```python
from build123d import *

# Parameters (mm, degrees)
SKICA1_R                 = 16.78
P_IDAT_VYSUNUT_M1_DEPTH  = 50.7
SKICA2_R                 = 5.65
P_IDAT_VYSUNUT_M2_DEPTH  = 4.61
SKICA3_R                 = 1.565
P_IDAT_VYSUNUT_M3_DEPTH  = 8.5
SKETCH6_R                = 23.5
BOSS_EXTRUDE1_DEPTH      = 3
SKETCH8_W                = 4.15
SKETCH8_H                = 3
SKETCH8_W_2              = 3
SKETCH8_H_2              = 4.15
ODEBRAT_VYSUNUT_M2_DEPTH = 3


with BuildPart() as part:
    # Skica1 → Přidat vysunutím1 (new body)
    with BuildSketch(Plane(origin=(0, 0, 0), x_dir=(1, 0, 0), z_dir=(0, 1, 0))):
        with Locations(Location((0, 0, 0), (0, 0, 90))):
            Circle(SKICA1_R)
    extrude(amount=P_IDAT_VYSUNUT_M1_DEPTH)

    # Skica2 → Přidat vysunutím2 (add)
    with BuildSketch(Plane(origin=(0, 50.7, 0), x_dir=(1, 0, 0), z_dir=(0, 1, 0))):
        with Locations(Location((0, 0, 0), (0, 0, 270))):
            Circle(SKICA2_R)
    extrude(amount=P_IDAT_VYSUNUT_M2_DEPTH)

    # Skica3 → Přidat vysunutím3 (add)
    with BuildSketch(Plane(origin=(0, 55.31, 0), x_dir=(1, 0, 0), z_dir=(0, 1, 0))):
        with Locations(Location((0, 0, 0), (0, 0, 270))):
            Circle(SKICA3_R)
    extrude(amount=P_IDAT_VYSUNUT_M3_DEPTH)

    # Sketch6 → Boss-Extrude1 (add)
    with BuildSketch(Plane.XZ):
        with Locations(Location((0, 0, 0), (0, 0, 270))):
            Circle(SKETCH6_R)
    extrude(amount=BOSS_EXTRUDE1_DEPTH)

    # Sketch8 → Odebrat vysunutím2 (cut)
    with BuildSketch(Plane(origin=(0, 0, 0), x_dir=(1, 0, 0), z_dir=(0, 1, 0))):
        with Locations((20.075, 0)):
            Rectangle(SKETCH8_W, SKETCH8_H)
        Polygon((11.66726189, -13.788582233), (14.601755032, -16.723075375), (16.723075375, -14.601755032), (13.788582233, -11.66726189), align=None)
        with Locations((0, -20.075)):
            Rectangle(SKETCH8_W_2, SKETCH8_H_2)
        Polygon((-13.788582233, -11.66726189), (-16.723075375, -14.601755032), (-14.601755032, -16.723075375), (-11.66726189, -13.788582233), align=None)
        with Locations((-20.075, 0)):
            Rectangle(SKETCH8_W, SKETCH8_H)
        Polygon((-11.66726189, 13.788582233), (-14.601755032, 16.723075375), (-16.723075375, 14.601755032), (-13.788582233, 11.66726189), align=None)
        with Locations((0, 20.075)):
            Rectangle(SKETCH8_W_2, SKETCH8_H_2)
        Polygon((13.788582233, 11.66726189), (16.723075375, 14.601755032), (14.601755032, 16.723075375), (11.66726189, 13.788582233), align=None)
        Polygon((6.151828996, -8.27314934), (9.086322138, -11.207642482), (11.207642482, -9.086322138), (8.27314934, -6.151828996), align=None)
        Polygon((-8.27314934, -6.151828996), (-11.207642482, -9.086322138), (-9.086322138, -11.207642482), (-6.151828996, -8.27314934), align=None)
        Polygon((-6.151828996, 8.27314934), (-9.086322138, 11.207642482), (-11.207642482, 9.086322138), (-8.27314934, 6.151828996), align=None)
        Polygon((8.27314934, 6.151828996), (11.207642482, 9.086322138), (9.086322138, 11.207642482), (6.151828996, 8.27314934), align=None)
    extrude(amount=-ODEBRAT_VYSUNUT_M2_DEPTH, mode=Mode.SUBTRACT)


solid = part.part
```
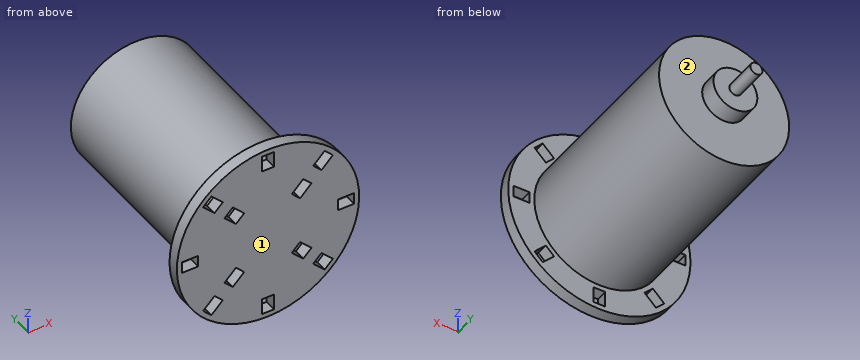
The listing builds one solid part. Answer for the finished solid, in the listing's coordinates (mm). Face numbers are marked on the shaded views. A direction names the side the tool comes from. Round coordinates to 2 decimals unless told otherwise and drop trailing zeros. Loops run counter-clockwise (first coordinate to the right, second up) from the corner with the lowest first, then second, coordinate; pieces in that order, holes last. Notation, with made-up numbers: (87, 74.5) -> (134, 74.5) arc R16 cw to (134, 79.5) -> close; hole circle Ø3 at (-14.75, 76.5). An arc over 180 degrees is marked (long way). Use one line per item in the form item = value.
1. The part is cut by section B-B on z = 0. Determine the outline of the cut face in (x, y) (3 decimals).
Answer key:
outline = (-23.5, -3) -> (-22.15, -3) -> (-22.15, 0) -> (-23.5, 0) -> close; (-18, -3) -> (18, -3) -> (18, 0) -> (16.78, 0) -> (16.78, 50.7) -> (5.65, 50.7) -> (5.65, 55.31) -> (1.565, 55.31) -> (1.565, 63.81) -> (-1.565, 63.81) -> (-1.565, 55.31) -> (-5.65, 55.31) -> (-5.65, 50.7) -> (-16.78, 50.7) -> (-16.78, 0) -> (-18, 0) -> close; (22.15, -3) -> (23.5, -3) -> (23.5, 0) -> (22.15, 0) -> close
2. A tool of negligible diameter and unlimited length cuts with its end or side. For the marked faces 1 and 2, from which of +Z, -Z, +X, -X, +Y, -Y can it reach the whole face along a straight path? Write none if from no direction.
Answer key:
face_1 = +Z, -Z, +X, -X, -Y
face_2 = +Y
3. The part is cut by section A-A on x = 0. Determine the outline of the cut face in (y, z) (3 decimals).
Answer key:
outline = (-3, -23.5) -> (0, -23.5) -> (0, -22.15) -> (-3, -22.15) -> close; (-3, -18) -> (0, -18) -> (0, -16.78) -> (50.7, -16.78) -> (50.7, -5.65) -> (55.31, -5.65) -> (55.31, -1.565) -> (63.81, -1.565) -> (63.81, 1.565) -> (55.31, 1.565) -> (55.31, 5.65) -> (50.7, 5.65) -> (50.7, 16.78) -> (0, 16.78) -> (0, 18) -> (-3, 18) -> close; (-3, 22.15) -> (0, 22.15) -> (0, 23.5) -> (-3, 23.5) -> close
4. Flat-ended cylindrical pins translate along their axes: pin 1 Ø3 at (x, z) = (-3.5, -17) entering from +Y; pin 2 Ø10 at (y, z) = (52.5, 4) entering from +X; pin 3 Ø1.5 at (x, y) = (20.5, -1) entering from -Z. Find the tip coordinate at first contact, or state that the pin passes through.
Answer key:
pin_1 = 50.7
pin_2 = 16.78
pin_3 = -12.74
5. Find the intervals of material crossed by probe 1 along Y at (x, z) = (-2, -20.5); probe 2 along X at (y, z) = (7.5, -12.5); probe 3 along Y at (x, z) = (-6, -14), in increasing order. Write a range as [from, to].
Answer key:
probe_1 = [-3, 0]
probe_2 = [-11.19, 11.19]
probe_3 = [-3, 50.7]
6. The part is cut by section C-C on z = -19. Determine the outline of the cut face in (x, y), and give its area (3 significant figures).
Answer key:
outline = (-13.83, -3) -> (-1.5, -3) -> (-1.5, 0) -> (-13.83, 0) -> close; (1.5, -3) -> (13.83, -3) -> (13.83, 0) -> (1.5, 0) -> close
area = 74.0 mm²
7. The part is cut by section D-D on y = 35.5. Determine the outline of the cut face in (x, z).
Answer key:
outline = circle Ø33.56 at (0, 0)
